Part model, mm, in its own coordinate system. Round coordinates to 2 decimals unless told otherwise and drop trailing zeros. Order: outer loops, then holes, each group sorted by start corner. A loop starts at its lowest first (then second) coordinate and runs counter-clockwise, first axis right, second up. Notation, with made-up numbers: (13.25, 28) -> (50.25, 28) arc R13 ccw to (50.25, 40) -> close; hole circle Ø1 at (-28.75, -40). An arc over 180 degrees is marked (long way). Return JSON: item names as keys, results as strings. Group by question number.
from build123d import *

# Parameters (mm, degrees)
SKETCH1_R           = 11
BOSS_EXTRUDE1_DEPTH = 5
SKETCH2_R           = 1.65
CUT_EXTRUDE2_DEPTH  = 21


with BuildPart() as part:
    # Sketch1 → Boss-Extrude1 (new body)
    with BuildSketch(Plane.XY):
        with Locations((-8.437318413, 0.250726348)):
            Circle(SKETCH1_R)
    extrude(amount=BOSS_EXTRUDE1_DEPTH)

    # Sketch2 → Cut-Extrude2 (cut)
    with BuildSketch(Plane.XY.offset(5)):
        with Locations((-8.437318413, 7.850726348)):
            Circle(SKETCH2_R)
        with Locations((-0.837318413, 0.250726348)):
            Circle(SKETCH2_R)
        with Locations((-8.437318413, -7.349273652)):
            Circle(SKETCH2_R)
        with Locations((-16.037318413, 0.250726348)):
            Circle(SKETCH2_R)
        with Locations((-8.437318413, 0.250726348)):
            Circle(SKETCH2_R)
    extrude(amount=-CUT_EXTRUDE2_DEPTH, mode=Mode.SUBTRACT)


solid = part.part
(1) Pin check, flat tips, straight feed: P1, Ø1, axis at y = 6, z = 0.5, coming from the -X side; P2, Ø1, axis at x = -12, z = 3.5, coming from the +Y side; P3, Ø1, axis at y = -6, z = 3.5, coming from the +X side. Stop position of each tip, or through.
(2) Mould opens along Y. For faces 1 (the cylindrical face through (-10.82, -10.49, 2.46)), 2 (the flat face through (-9, -2, 5)), 3 (the cylindrical face through (-17.35, -0.75, 2.54)) say: pulls with the +Y half, pulls with the -Y half, needs draft (parallel to the pull), parting line crosses it, or undercut.
(3) Saw through at B-B, the plane y = -7.75. List the corners of the cut face in (x, z), and give its area (3 significant figures).
(4) Saw through at A-A, the plane x = -16.5. List the corners of the cut face in (y, z), and give its area (3 significant figures).
(5) Saw through at D-D, the plane z = 3.9. List the corners of the cut face in (x, y).
(6) Saw through at C-C, the plane x = -8.5. List the corners of the cut face in (y, z).
(7) Probe L1, parallel to X at y = 0, z = 1.95; L2, parallel to Y at x = -9.25, z = 3.8; L3, parallel to Y at x = -7.5, z = 0.55. List the from-to ranges inside material, lowest first. Write a range as [from, to].
Results are:
{
 "1": {"P1": "stops at x = -18.1", "P2": "stops at y = 10.82", "P3": "stops at x = 0.94"},
 "2": {"face 1": "parting line crosses it", "face 2": "needs draft", "face 3": "undercut"},
 "3": {"outline": "(-15.99, 0) -> (-10.04, 0) -> (-10.04, 5) -> (-15.99, 5) -> close; (-6.84, 0) -> (-0.89, 0) -> (-0.89, 5) -> (-6.84, 5) -> close", "area": "59.5 mm^2"},
 "4": {"outline": "(-7.23, 0) -> (-1.33, 0) -> (-1.33, 5) -> (-7.23, 5) -> close; (1.83, 0) -> (7.73, 0) -> (7.73, 5) -> (1.83, 5) -> close", "area": "59.0 mm^2"},
 "5": {"outline": "circle Ø22 at (-8.44, 0.25); hole circle Ø3.3 at (-16.04, 0.25); hole circle Ø3.3 at (-8.44, -7.35); hole circle Ø3.3 at (-8.44, 0.25); hole circle Ø3.3 at (-8.44, 7.85); hole circle Ø3.3 at (-0.84, 0.25)"},
 "6": {"outline": "(-10.75, 0) -> (-9, 0) -> (-9, 5) -> (-10.75, 5) -> close; (-5.7, 0) -> (-1.4, 0) -> (-1.4, 5) -> (-5.7, 5) -> close; (1.9, 0) -> (6.2, 0) -> (6.2, 5) -> (1.9, 5) -> close; (9.5, 0) -> (11.25, 0) -> (11.25, 5) -> (9.5, 5) -> close"},
 "7": {"L1": "x = [-19.43, -17.67], [-14.41, -10.07], [-6.81, -2.47], [0.79, 2.56]", "L2": "y = [-10.72, -8.79], [-5.91, -1.19], [1.69, 6.41], [9.29, 11.22]", "L3": "y = [-10.71, -8.71], [-5.99, -1.11], [1.61, 6.49], [9.21, 11.21]"}
}
